Geometry check sheet. Reference: drawing and pictorial views, mm from the part's lowest x, y, z. A direction names the side the tool comes from. Round coordinates to 2 decimals unless told otherwise and drop trailing zeros. Write each loop counter-clockwise with the first axis right and the second up, starting at its lowest first coordinate (ties: lowest second). Pieces come first, ordered by that corner, then holes. Notation, with made-up numbers: (-12, 42) -> (-2, 42) arc R26 cw to (-2, 59) -> close; hole circle Ø10 at (34, 62.25). An arc over 180 degrees is marked (long way). Write item = value, one per line.
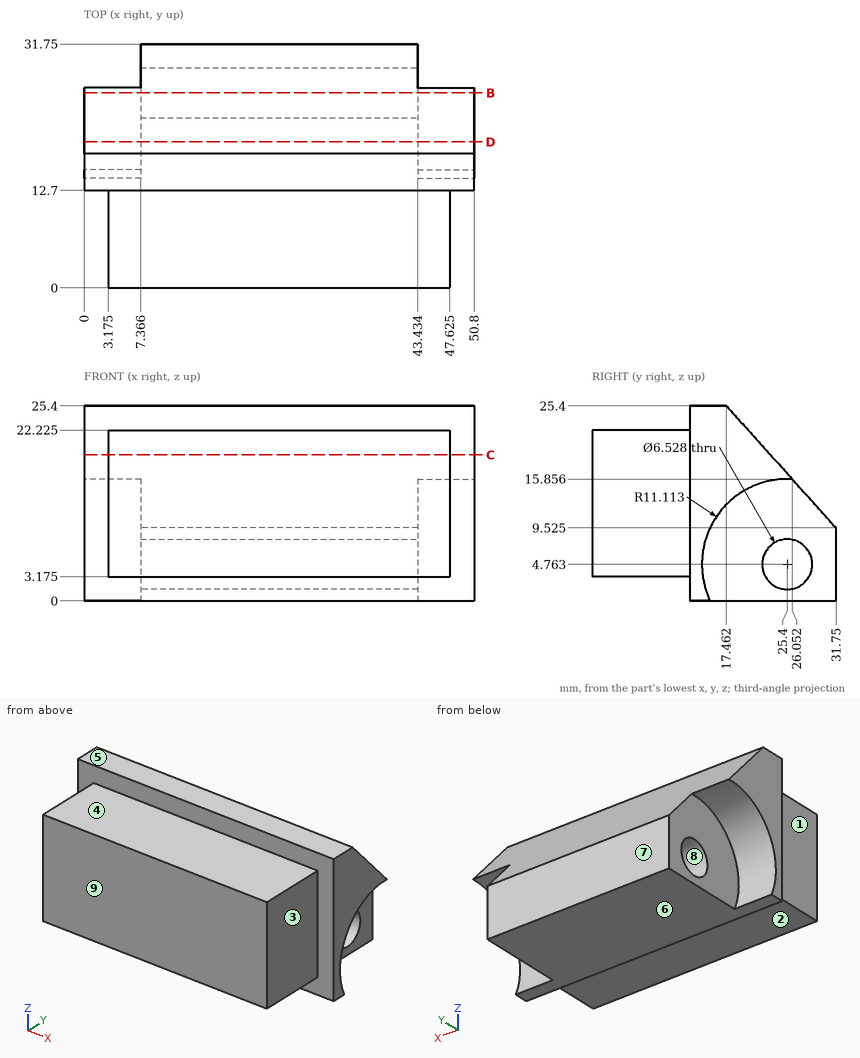
(1) Release check for a two-part mould opening along Y. For the marked faces 6, 7, 8 and 9 record: pulls with the +Y half, pulls with the -Y half, needs draft (parallel to the pull), parting line crosses it, or undercut.
Worked answers:
face_6 = needs draft
face_7 = pulls with the +Y half
face_8 = undercut
face_9 = pulls with the -Y half
(2) Sectioned sample at C-C on z = 19. Enter the section's corners in (x, y) (1 decimal).
Worked answers:
outline = (0, 12.7) -> (3.2, 12.7) -> (3.2, 0) -> (47.6, 0) -> (47.6, 12.7) -> (50.8, 12.7) -> (50.8, 23.2) -> (0, 23.2) -> close
(3) Sectioned sample at B-B on y = 25.4. Enter the section's corners in (x, z) (1 decimal).
Worked answers:
outline = (0, 15.9) -> (7.4, 15.9) -> (7.4, 8) -> (43.4, 8) -> (43.4, 15.9) -> (50.8, 15.9) -> (50.8, 16.6) -> (0, 16.6) -> close; (7.4, 0) -> (43.4, 0) -> (43.4, 1.5) -> (7.4, 1.5) -> close
(4) Sectioned sample at D-D on y = 19. Enter the section's corners in (x, z) (1 decimal).
Worked answers:
outline = (0, 13.8) -> (7.4, 13.8) -> (7.4, 0) -> (43.4, 0) -> (43.4, 13.8) -> (50.8, 13.8) -> (50.8, 23.7) -> (0, 23.7) -> close
(5) Go/stop test with flat-tipped pins: P1, Ø2, axis at y = 26.5, z = 12.5, coming from the -X side; P2, Ø4, axis at y = 9.5, z = 13, coming from the -X side (1 decimal); P3, Ø1, axis at x = 31, y = 25, coming from the +Z side; P4, Ø4, axis at y = 25.4, z = 4.76, coming from the +X side. Record where each tip stops, or that it passes through.
Worked answers:
P1 = 7.37
P2 = 3.2
P3 = 17.58
P4 = through
(6) Access from +Z, -Z, +X, -X, +Y, -Y to the whole of each face (thin tool, end or side, straight path). Record for the marked faces 1, 2, 3, 4 and 5.
Worked answers:
face_1 = +Z, -Z, -X, -Y
face_2 = -Z, +X, -X, -Y
face_3 = +Z, -Z, +X, -Y
face_4 = +Z, +X, -X, -Y
face_5 = +Z, +X, -X, +Y, -Y
(7) Material ranges on L1, parallel to X at y = 5, z = 18.5 (1 decimal); L2, parallel to X at y = 17, z = 5.25 (1 decimal); L3, parallel to Z at x = 26.5, y = 12 (1 decimal), recorded low to high. Write a range as [from, to].
Worked answers:
L1 = [3.2, 47.6]
L2 = [7.4, 43.4]
L3 = [3.2, 22.2]
